For this review, take the finished solid that the model builds, in its own axes (mm). Face numbers are marked on the shaded views. Round coordinates to 2 decimals unless told otherwise and drop trailing zeros. Write each loop counter-clockwise with the first axis right and the second up, starting at its lowest first coordinate (ties: lowest second). Pieces come first, ordered by that corner, then holes. Notation, with made-up numbers: M -13.75,1 L -2.75,1 A17 ccw -2.75,24 Z; hole C 84.25,26.25 d10. An arc over 180 degrees is marked long. One line per question, with ' | ' between items.
```python
from build123d import *

# Parameters (mm, degrees)
PAD_DEPTH    = 20
PAD001_DEPTH = 20


with BuildPart() as part:
    # Sketch001 → Pad (new body)
    with BuildSketch(Plane.XY):
        with BuildLine():
            ThreePointArc((3.462658, -4.9), (5.718391, 1.81659), (0, 6))
            Line((0, 6), (0, 9))
            ThreePointArc((0, -9), (9, 0), (0, 9))
            Line((0, -4.9), (0, -9))
            Line((3.462658, -4.9), (0, -4.9))
        make_face()
    pad = extrude(amount=PAD_DEPTH)

    # Sketch002 → Pad001 (join)
    with BuildSketch(Plane.XY):
        with BuildLine():
            ThreePointArc((2.12132, -3.45), (3.897114, 1.10227), (0, 4.05))
            Line((0, 4.05), (0, 9))
            ThreePointArc((0, -9), (9, 0), (0, 9))
            Line((0, -3.45), (0, -9))
            Line((2.12132, -3.45), (0, -3.45))
        make_face()
    pad001 = extrude(amount=-PAD001_DEPTH)

    # Mirrored: Pad, Pad001 across Sketch001 V_Axis
    add(pad.mirror(Plane(origin=(0, 0, 0), x_dir=(0, 0, 1), z_dir=(1, 0, 0))))
    add(pad001.mirror(Plane(origin=(0, 0, 0), x_dir=(0, 0, 1), z_dir=(1, 0, 0))))


solid = part.part
```
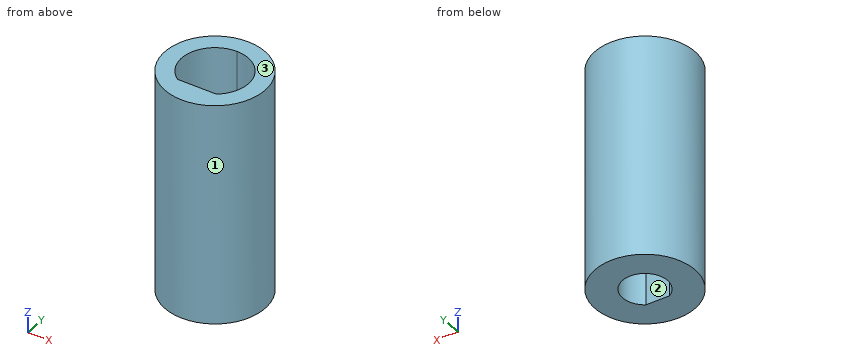
Item 1: Take a section at B-B (z = 6.5). Write out the cut boundary in (x, y).
Results:
outline: C 0,0 d18; hole M -3.46,-4.9 L 3.46,-4.9 A6 ccw 0,6 A6 ccw Z
Item 2: To check wall thickness, follow line 1 along X through (y, z) = (0.25, -17.5); line 2 along X through (y, z) = (2.75, 7); line 3 along Z through (x, y) = (0.75, -3.5). State the ranges of each line that lie inside material, in increasing order. Write a range as from..to.
Results:
line 1: -9..-4.04, 4.04..9 | line 2: -8.57..-5.33, 5.33..8.57 | line 3: -20..0
Item 3: Take a section at C-C (x = -5.5). Write out the cut boundary in (y, z), then the cut area to 3 significant figures.
Results:
outline: M -7.12,-20 L 7.12,-20 L 7.12,20 L 2.4,20 L 2.4,0 L -2.4,0 L -2.4,20 L -7.12,20 Z | area: 474 mm2
Item 4: Insertion check: pin 1 Ø6 at (x, y) = (2.5, -4.5) entering from +Z; pin 2 Ø1.5 at (x, z) = (-4.5, 14) entering from -Y; pin 3 Ø8 at (y, z) = (-5.5, 8) entering from +X; pin 4 Ø4 at (y, z) = (-6.5, 2.5) entering from -X. Each pin has a flat end and moves straight along its axis. Give the tip position at first contact, or say it passes through.
Results:
pin 1: z = 20 | pin 2: y = -8.18 | pin 3: x = 8.87 | pin 4: x = -7.79
Item 5: Mouldability with a two-part tool opening along X and no side actions: class the marked faces 1, 2 and 3 as +X half, -X half, draft (parallel to the pull), parting line (faces both ways), or undercut.
Results:
face 1: parting line | face 2: undercut | face 3: draft
Item 6: Take a section at A-A (y = 0). Write out the cut boundary in (x, z).
Results:
outline: M -9,-20 L -4.05,-20 L -4.05,0 L -6,0 L -6,20 L -9,20 Z; M 4.05,-20 L 9,-20 L 9,20 L 6,20 L 6,0 L 4.05,0 Z
Item 7: Take a section at D-D (y = 3.5). Write out the cut boundary in (x, z), then the cut area to 3 significant figures.
Results:
outline: M -8.29,-20 L -2.04,-20 L -2.04,0 L -4.87,0 L -4.87,20 L -8.29,20 Z; M 2.04,-20 L 8.29,-20 L 8.29,20 L 4.87,20 L 4.87,0 L 2.04,0 Z | area: 387 mm2
